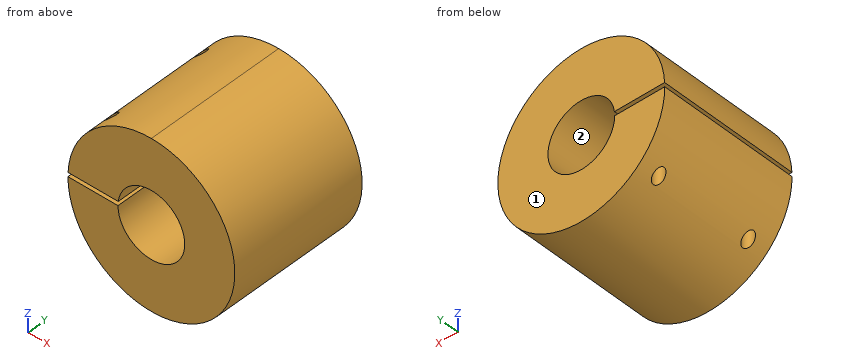
```python
from build123d import *

# Parameters (mm, degrees)
SKETCH1_R               = 25.4
BOSS_EXTRUDE1_DEPTH     = 42.799
CUT_EXTRUDE1_DEPTH      = 56.875525957
CUT_EXTRUDE2_DEPTH      = 72.116484735
CUT_EXTRUDE2_DEPTH_BACK = 72.116484735
SKETCH3_R               = 1.651


with BuildPart() as part:
    # Sketch1 → Boss-Extrude1 (new body)
    with BuildSketch(Plane(origin=(0, 0, 0), x_dir=(1, 0, 0), z_dir=(0, 1, 0))):
        with Locations(Location((0, 0, 0), (0, 0, 270))):
            Circle(SKETCH1_R)
    extrude(amount=BOSS_EXTRUDE1_DEPTH)

    # Sketch2 → Cut-Extrude1 (cut, through all)
    with BuildSketch(Plane(origin=(0, 42.799, 0), x_dir=(1, 0, 0), z_dir=(0, 1, 0))):
        with BuildLine():
            Line((-10.16, 0), (-25.4, 0))
            ThreePointArc((-25.4, 0), (-25.392056291, -0.635198655), (-25.368230131, -1.27))
            Line((-25.368230131, -1.27), (-10.080312495, -1.27))
            ThreePointArc((-10.080312495, -1.27), (10.140058554, 0.636248791), (-10.16, 0))
        make_face()
    extrude(amount=-CUT_EXTRUDE1_DEPTH, mode=Mode.SUBTRACT)

    # Sketch3 → Cut-Extrude2 (cut, two sides: drawn at the far end of the back side and taken through both)
    with BuildSketch(Plane.XY.offset(-25.4).offset(-CUT_EXTRUDE2_DEPTH_BACK)):
        with Locations(Location((-17.78, 36.449, 0), (0, 0, 180))):
            Circle(SKETCH3_R)
        with Locations(Location((-17.78, 6.35, 0), (0, 0, 180))):
            Circle(SKETCH3_R)
    extrude(amount=CUT_EXTRUDE2_DEPTH + CUT_EXTRUDE2_DEPTH_BACK, mode=Mode.SUBTRACT)


solid = part.part
```
Read the model definition and answer for the solid it produces. Units are mm, in the model's axes. Face numbers are marked on the shaded views. Coordinates: 2 decimals unless noted, no trailing zeros. Write each loop counter-clockwise with the first axis right and the second up, starting at its lowest first coordinate (ties: lowest second). Pieces come first, ordered by that corner, then holes. Notation, with made-up numbers: (56, -16) - (102, -16) arc R23 cw to (102, 21) - close; hole circle Ø11 at (71.5, 85). An arc over 180 degrees is marked (long way). Answer as a JSON object with one key per item and string values. Group by question number.
1. A cutting plane is placed at A-A (x = -17.78). Determine the outline of the cut face in (y, z), plus the area to 3 significant figures.
2. The mould has two halves that part along Z. Classify the marked faces 1 and 2: +Z half, -Z half, draft (parallel to the pull), parting line (faces both ways), or undercut.
3. Each of these flat-tipped pins is pushed along its axis until it touches: P1, Ø12, axis at x = 0, z = 0, coming from the +Y side; P2, Ø17, axis at x = -19, y = 22, coming from the -Z side; P3, Ø12, axis at x = -15.5, y = 25.5, coming from the +Z side; P4, Ø1.5, axis at x = -2.5, y = 14.5, coming from the +Z side. Where does it stop, or does it pass through?
4. A cutting plane is placed at D-D (x = 9). Determine the outline of the cut face in (y, z), plus the area to 3 significant figures.
5. Consider L1, parallel to Y at x = -17.78, z = -11.25; L2, parallel to X at y = 5.5, z = -3.5; L3, parallel to Z at x = 0, y = 30. Determine where each line is inside the solid, lowest interval first. Write a range as [from, to].
6. A cutting plane is placed at C-C (z = -11.5). Determine the outline of the cut face in (x, y).
7. A cutting plane is placed at B-B (y = 6.35). Determine the outline of the cut face in (x, z), plus the area to 3 significant figures.
Worked out:
{
 "1": {"outline": "(0, -18.14) - (4.7, -18.14) - (4.7, 0) - (0, 0) - close; (0, 1.27) - (4.7, 1.27) - (4.7, 18.14) - (0, 18.14) - close; (8, -18.14) - (34.8, -18.14) - (34.8, 0) - (8, 0) - close; (8, 1.27) - (34.8, 1.27) - (34.8, 18.14) - (8, 18.14) - close; (38.1, -18.14) - (42.8, -18.14) - (42.8, 0) - (38.1, 0) - close; (38.1, 1.27) - (42.8, 1.27) - (42.8, 18.14) - (38.1, 18.14) - close", "area": "1,270 mm²"},
 "2": {"face 1": "draft", "face 2": "undercut"},
 "3": {"P1": "passes through", "P2": "stops at z = -23.13", "P3": "stops at z = 23.56", "P4": "stops at z = 25.34"},
 "4": {"outline": "(0, -23.75) - (42.8, -23.75) - (42.8, -4.71) - (0, -4.71) - close; (0, 4.71) - (42.8, 4.71) - (42.8, 23.75) - (0, 23.75) - close", "area": "1,630 mm²"},
 "5": {"L1": "y = [0, 4.7], [8, 34.8], [38.1, 42.8]", "L2": "x = [-25.16, -19.2], [-16.36, -9.54], [9.54, 25.16]", "L3": "z = [-25.4, -10.16], [10.16, 25.4]"},
 "6": {"outline": "(-22.65, 0) - (22.65, 0) - (22.65, 42.8) - (-22.65, 42.8) - close; hole circle Ø3.3 at (-17.78, 6.35); hole circle Ø3.3 at (-17.78, 36.45)"},
 "7": {"outline": "(-25.4, 0) arc R25.4 ccw to (-19.43, -16.36) - (-19.43, 0) - close; (-25.37, 1.27) - (-19.43, 1.27) - (-19.43, 16.36) arc R25.4 ccw to start; (-16.13, -19.62) arc R25.4 ccw (long way) to (-16.13, 19.62) - (-16.13, 1.27) - (-10.08, 1.27) arc R10.16 cw (long way) to (-10.16, 0) - (-16.13, 0) - close", "area": "1,570 mm²"}
}
